For this review, take the finished solid that the model builds, in its own axes (mm). Round coordinates to 2 decimals unless told otherwise and drop trailing zeros. Write each loop counter-clockwise with the first axis right and the second up, starting at its lowest first coordinate (ties: lowest second). Pieces come first, ordered by that corner, then holes. Notation, with made-up numbers: M 55,-25 L 95,-25 A27 cw 95,5 Z; hole C 36,13.25 d6. An arc over 180 degrees is marked long. Write each question's results on one line, items separated by ' | '. Start each with the question number.
```python
from build123d import *

# Parameters (mm, degrees)
EXTRUDE_1_DEPTH   = 2
HOLE_WIZARD_M61_D = 6.6
CHAMFER_1_SIZE    = 2.5


with BuildPart() as part:
    # Эскиз3 → Бобышка-Вытянуть1 (new body)
    with BuildSketch(Plane(origin=(0, 0, 0), x_dir=(1, 0, 0), z_dir=(0, 0, -1))):
        Polygon((0, 0), (75, 0), (75, 119.903810568), (49.019237886, 134.903810568), (0, 50), align=None)
    extrude(amount=EXTRUDE_1_DEPTH)

    # Отверстие с зазором M61 (through all)
    with Locations(Plane(origin=(0, 0, -2), x_dir=(1, 0, 0), z_dir=(0, 0, -1))):
        with Locations((15, 15), (60, 15), (20, 54.641016151), (54.509618943, 114.413429511)):
            Hole(HOLE_WIZARD_M61_D / 2)

    # Фаска1
    chamfer_1_edges = [part.edges().sort_by_distance(p)[0] for p in [
        (49.019237886, -134.903810568, -1),
        (75, 0, -1),
        (0, 0, -1),
    ]]
    chamfer(chamfer_1_edges, length=CHAMFER_1_SIZE)


solid = part.part
```
Item 1: Mouldability with a two-part tool opening along Y and no side actions: class faces 1 (the cylindrical face through (54.939, -117.685, -0.986)), 2 (the flat face through (1.2, -1.3, -1)), 3 (the cylindrical face through (18.226, -57.424, -0.986)), 4 (the flat face through (45, -53, -2)) as pulls with the +Y half, pulls with the -Y half, needs draft (parallel to the pull), parting line crosses it, or undercut.
Item 2: We need section D-D on z = -0.85. State the section outline as (x, y) points, then the cut area to 3 significant figures.
Item 3: We need section C-C on y = -116. State the section outline as (x, z) points.
Item 4: We need section B-B on x = 60. State the section outline as (y, z) points.
Item 5: For probe 1 along X at (y, z) = (-113.5, -1.1); probe 2 along Y at (x, z) = (20, -1.45); probe 3 along X at (y, z) = (-53, -1.9), list the stretches that pass through material, from the lowest coordinate up.
Item 6: We need section A-A on y = -15. State the section outline as (x, z) points.
Numbers:
1) face 1: undercut | face 2: pulls with the +Y half | face 3: undercut | face 4: needs draft
2) outline: M 0,-50 L 47.77,-132.74 L 51.18,-133.65 L 75,-119.9 L 75,-2.5 L 72.5,0 L 2.5,0 L 0,-2.5 Z; hole C 15,-15 d6.6; hole C 20,-54.64 d6.6; hole C 54.51,-114.41 d6.6; hole C 60,-15 d6.6 | area: 7,700 mm^2
3) outline: M 38.11,-2 L 51.62,-2 L 51.62,0 L 38.11,0 Z; M 57.4,-2 L 75,-2 L 75,0 L 57.4,0 Z
4) outline: M -128.56,-2 L -18.3,-2 L -18.3,0 L -128.56,0 Z; M -11.7,-2 L 0,-2 L 0,0 L -11.7,0 Z
5) probe 1: x = 36.66 to 51.34, 57.68 to 75 | probe 2: y = -84.64 to -57.94, -51.34 to 0 | probe 3: x = 1.73 to 17.14, 22.86 to 75
6) outline: M 0,-2 L 11.7,-2 L 11.7,0 L 0,0 Z; M 18.3,-2 L 56.7,-2 L 56.7,0 L 18.3,0 Z; M 63.3,-2 L 75,-2 L 75,0 L 63.3,0 Z
